Geometry check sheet. Reference: the model listing, model coordinates, mm. A direction names the side the tool comes from. Give positions to 0.01 mm unless a question says otherwise; leave off trailing zeros. Write each loop counter-clockwise with the first axis right and the second up, starting at its lowest first coordinate (ties: lowest second). Pieces come first, ordered by that corner, then holes. Notation, with made-up numbers: M -11,40 L 6,40 A7 ccw 6,44 Z; hole C 68.25,-19.5 d2. An arc over 180 degrees is marked long. One line per item, written item: value. Start each with the question number.
1. Cross-section at A-A on z = 0. Record the cut outline in (x, y).
2. Tool access check on faces 4 (the face through (-56, 3, -211.528)), 5 (the face through (7.78, 3.131, 24.704)), 6 (the face through (56, 3, -218.672)). Record the directions out of +Z, -Z, +X, -X, +Y, -Y that give a thin tool (end or side, any length) a straight path to the whole face; none if there is none.
3. Cross-section at D-D on z = -215.1. Record the cut outline in (x, y).
4. Release check for a two-part mould opening along Z. For faces 1 (the face through (-63.5, 3, -2)), 2 (the face through (56, 3, -33.728)), 3 (the face through (-60.65, 3.22, 32.99)) record: pulls with the +Z half, pulls with the -Z half, needs draft (parallel to the pull), parting line crosses it, or undercut.
5. Cross-section at C-C on x = 0. Record the cut outline in (y, z).
6. Scan lines: line 1 (X direction, y = 2.75, z = 0); line 2 (Z direction, x = -1.5, y = 5.75); line 3 (Z direction, x = 22, y = 1.75). Record each from-to range of solid material in increasing order.
7. Gauge pin test, flat ends, axial feed: pin 1 (3 mm diameter, centred on x = -56.5, y = 2.5, fed in from -Z); pin 2 (1.9 mm diameter, centred on x = -56, y = 3, fed in from +Z); pin 3 (1.9 mm diameter, centred on x = -58.5, y = 4.5, fed in from -Z). Record the tip position at first contact, or that the pin passes through.
from build123d import *

# Parameters (mm, degrees)
SKETCH1_W           = 127
SKETCH1_H           = 289.2
SKETCH1_R           = 25.9
BOSS_EXTRUDE1_DEPTH = 6.35
CUT_EXTRUDE1_DEPTH  = 7.35
FILLET1_R           = 2
FILLET2_R           = 10


with BuildPart() as part:
    # Sketch1 → Boss-Extrude1 (new body)
    with BuildSketch(Plane(origin=(0, 0, 0), x_dir=(1, 0, 0), z_dir=(0, 1, 0))):
        with Locations((0, 108.6)):
            Rectangle(SKETCH1_W, SKETCH1_H)
        with Locations(Location((0, 0, 0), (0, 0, 270))):  # turned: the seam where the file's is
            Circle(SKETCH1_R, mode=Mode.SUBTRACT)
    extrude(amount=BOSS_EXTRUDE1_DEPTH)

    # Sketch3 → Cut-Extrude1 (cut, through all)
    with BuildSketch(Plane(origin=(0, 6.35, 0), x_dir=(1, 0, 0), z_dir=(0, 1, 0))):
        with BuildLine():
            Line((-76.2, 218.671875), (-50.8, 218.671875))
            ThreePointArc((-50.8, 218.671875), (-47.228125, 215.1), (-50.8, 211.528125))
            Line((-50.8, 211.528125), (-76.2, 211.528125))
            ThreePointArc((-76.2, 211.528125), (-79.771875, 215.1), (-76.2, 218.671875))
        make_face()
        with BuildLine():
            Line((-76.2, 40.871875), (-50.8, 40.871875))
            ThreePointArc((-50.8, 40.871875), (-47.228125, 37.3), (-50.8, 33.728125))
            Line((-50.8, 33.728125), (-76.2, 33.728125))
            ThreePointArc((-76.2, 33.728125), (-79.771875, 37.3), (-76.2, 40.871875))
        make_face()
    cut_extrude1 = extrude(amount=-CUT_EXTRUDE1_DEPTH, mode=Mode.SUBTRACT)

    # Mirror1: Cut-Extrude1 across plane
    add(cut_extrude1.mirror(Plane(origin=(0, 0, 0), x_dir=(0, 0, 1), z_dir=(1, 0, 0))), mode=Mode.SUBTRACT)

    # Fillet1
    fillet1_edges = [part.edges().sort_by_distance(p)[0] for p in [
        (-63.5, 3.175, -211.528125),
        (-63.5, 3.175, -218.671875),
        (-63.5, 3.175, -40.871875),
        (-63.5, 3.175, -33.728125),
        (63.5, 3.175, -218.671875),
        (63.5, 3.175, -211.528125),
        (63.5, 3.175, -33.728125),
        (63.5, 3.175, -40.871875),
    ]]
    fillet(fillet1_edges, radius=FILLET1_R)

    # Fillet2
    fillet2_edges = [part.edges().sort_by_distance(p)[0] for p in [
        (-63.5, 3.175, -253.2),
        (63.5, 3.175, -253.2),
        (63.5, 3.175, 36),
        (-63.5, 3.175, 36),
    ]]
    fillet(fillet2_edges, radius=FILLET2_R)


solid = part.part
Report:
1. outline: M -63.5,0 L -25.9,0 L -25.9,6.35 L -63.5,6.35 Z; M 25.9,0 L 63.5,0 L 63.5,6.35 L 25.9,6.35 Z
2. face 4: -X, +Y, -Y
2. face 5: +Y, -Y
2. face 6: +X, +Y, -Y
3. outline: M -47.23,0 L 47.23,0 L 47.23,6.35 L -47.23,6.35 Z
4. face 1: needs draft
4. face 2: undercut
4. face 3: pulls with the +Z half
5. outline: M 0,-253.2 L 6.35,-253.2 L 6.35,-25.9 L 0,-25.9 Z; M 0,25.9 L 6.35,25.9 L 6.35,36 L 0,36 Z
6. line 1: x = -63.5 to -25.9, 25.9 to 63.5
6. line 2: z = -253.2 to -25.86, 25.86 to 36
6. line 3: z = -253.2 to -13.67, 13.67 to 36
7. pin 1: stops at z = -253.09
7. pin 2: stops at z = 35.88
7. pin 3: stops at z = -252.34
